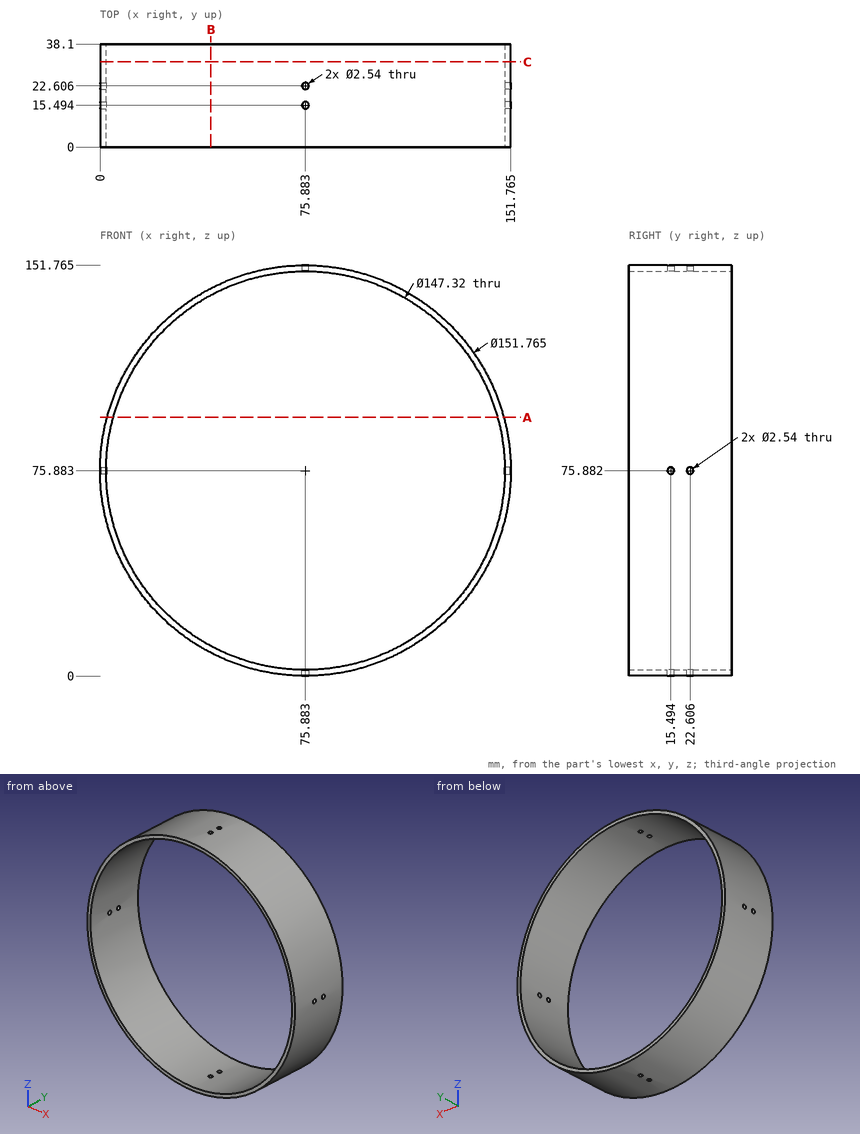
Answer from the drawing. Dimensions are ordinates in mm from the lowest x, y and z of the part. Coordinates: 2 decimals unless noted, no trailing zeros. Write each loop counter-clockwise with the first axis right and the second up, starting at its lowest first coordinate (ties: lowest second). Pieces come first, ordered by that corner, then holes. Notation, with made-up numbers: (19, 67) - (40, 67) arc R18 cw to (40, 100) - close; hole circle Ø7 at (24, -37.75). An arc over 180 degrees is marked (long way). Return JSON: item names as keys, results as strings. Group by question number.
Q1. Flat-ended cylindrical pins translate along their axes: pin 1 Ø8 at (x, z) = (20, 29) entering from -Y; pin 2 Ø12 at (y, z) = (30.5, 111.5) entering from +X; pin 3 Ø1.5 at (x, y) = (20, 21.5) entering from -Z; pin 4 Ø12 at (x, y) = (132.5, 12) entering from -Z. Find the tip coordinate at first contact, or state that the pin passes through.
Q2. The part is cut by section A-A on z = 95.5. Write down the section's boundary in (x, y) (1 decimal).
Q3. The part is cut by section C-C on y = 31.5. Write down the section's boundary in (x, z) (1 decimal).
Q4. The part is cut by section B-B on x = 41. Write down the section's boundary in (y, z) (1 decimal).
Q5. Find the intervals of material crossed by line 1 along Z through (x, y) = (21.5, 6) (1 decimal); line 2 along X through (y, z) = (21, 73) (1 decimal); line 3 along Z through (x, y) = (35.5, 26.5) (1 decimal), in increasing order. Write a range as [from, to].
Evaluation:
{
 "1": {"pin 1": "stops at y = 0", "pin 2": "stops at x = 145.75", "pin 3": "stops at z = 23.74", "pin 4": "stops at z = 19.35"},
 "2": {"outline": "(2.6, 0) - (4.9, 0) - (4.9, 38.1) - (2.6, 38.1) - close; (146.9, 0) - (149.2, 0) - (149.2, 38.1) - (146.9, 38.1) - close"},
 "3": {"outline": "circle Ø151.8 at (75.9, 75.9); hole circle Ø147.3 at (75.9, 75.9)"},
 "4": {"outline": "(0, 8.5) - (38.1, 8.5) - (38.1, 11) - (0, 11) - close; (0, 140.8) - (38.1, 140.8) - (38.1, 143.3) - (0, 143.3) - close"},
 "5": {"line 1": "z = [23, 26.2], [125.6, 128.8]", "line 2": "x = [0.1, 2.3], [149.5, 151.7]", "line 3": "z = [11.6, 14.3], [137.5, 140.1]"}
}
